For this review, take the finished solid that the model builds, in its own axes (mm). A direction names the side the tool comes from. Coordinates: 2 decimals unless noted, no trailing zeros. Loops run counter-clockwise (first coordinate to the right, second up) from the corner with the lowest first, then second, coordinate; pieces in that order, holes last. Notation, with made-up numbers: M 43.25,84.5 L 101.25,84.5 A22 cw 101.25,107.5 Z; hole C -26,-15 d7. An arc over 180 degrees is marked long. Answer as a JSON object with one key per item and string values. Group by question number.
Item 1: Add section D-D (x = 3.5). State the section outline as (y, z) points, then the cut area to 3 significant figures.
Item 2: Insertion check: pin 1 (10 mm diameter, centred on y = -0.5, z = 0, fed in from +X); pin 2 (1 mm diameter, centred on x = 3, z = -6, fed in from -Y); pin 3 (3 mm diameter, centred on x = 6, y = 1, fed in from -Z); pin 4 (1.9 mm diameter, centred on x = 5.5, y = 0, fed in from -Z). Each pin has a flat end and moves straight along its axis. Give the tip position at first contact, or say it passes through.
Item 3: Add section C-C (z = 5.5). State the section outline as (x, y) points.
Item 4: Add section A-A (x = 5.5). State the section outline as (y, z) points, then the cut area to 3 significant figures.
Item 5: Add section B-B (y = 0). State the section outline as (x, z) points.
Item 6: Mouldability with a two-part tool opening along Y and no side actions: class faces 1 (the face through (1.5, -16.5, 0.1)), 2 (the face through (1, -17.5, 0)), 3 (the face through (7.4, 5.93, -5.49)), 4 (the face through (3.6, -0.1, 4.5)) as +Y half, -Y half, draft (parallel to the pull), parting line (faces both ways), or undercut.
Item 7: Wall thickness on L1, parallel to Z at x = 5, y = 2.5; L2, parallel to Y at x = 5.5, z = 6; L3, parallel to X at y = 13, z = 7: over which ranges is each line inside the solid? List them lowest first. Write a range as from..to.
Item 8: Tool access review of faces 5 (the face through (3.6, -0.1, -6.5)), 6 (the face through (5, 6.5, -6)), 7 (the face through (1.5, -15.5, 7.5)), 8 (the face through (3.6, -0.1, -4.5)), 9 (the face through (5, -6.5, 5)): name each direction out of +Z, -Z, +X, -X, +Y, -Y from which nothing blocks a thin tool from reaching the whole face with its end or side.
from build123d import *

# Parameters (mm, degrees)
F0_W     = 35
F0_H     = 17
F1_DEPTH = 2
F2_W     = 2
F2_H     = 13
F2_H_2   = 1
F3_DEPTH = 1
F4_W     = 13
F4_H     = 2
F5_DEPTH = 6
F7_D     = 3.2
F8_R     = 2


with BuildPart() as f1:
    # F0 (on Right) → F1 (new body)
    with BuildSketch(Plane.YZ):
        Rectangle(F0_W, F0_H)
    extrude(amount=F1_DEPTH)

    # F2 (on face) → F3 (cut)
    with BuildSketch(Plane.YZ.offset(2)):
        with Locations((-15.5, 0)):
            Rectangle(F2_W, F2_H)
        with Locations((-15.5, 7)):
            Rectangle(F2_W, F2_H_2)
        with Locations((-15.5, -7)):
            Rectangle(F2_W, F2_H_2)
    extrude(amount=-F3_DEPTH, mode=Mode.SUBTRACT)

    # F4 (on face) → F5 (join)
    with BuildSketch(Plane.YZ.offset(2)):
        with Locations((0, 5.5)):
            Rectangle(F4_W, F4_H)
        with Locations((0, -5.5)):
            Rectangle(F4_W, F4_H)
    extrude(amount=F5_DEPTH)

    # F7 (through all)
    with Locations(Plane.XY.offset(6.5)):
        with Locations((5.5, 0)):
            Hole(F7_D / 2)

    # F8
    f8_edges = [f1.edges().sort_by_distance(p)[0] for p in [
        (2, 6.5, 5.5),
        (8, 6.5, 5.5),
        (8, 6.5, -5.5),
        (2, 6.5, -5.5),
        (2, -6.5, -5.5),
        (8, -6.5, -5.5),
        (2, -6.5, 5.5),
        (8, -6.5, 5.5),
    ]]
    fillet(f8_edges, radius=F8_R)


solid = f1.part
From the geometry:
{
 "1": {"outline": "M -6.56,-6.5 L 6.56,-6.5 L 6.56,-4.5 L -6.56,-4.5 Z; M -6.56,4.5 L 6.56,4.5 L 6.56,6.5 L -6.56,6.5 Z", "area": "52.5 mm²"},
 "2": {"pin 1": "stops at x = 8", "pin 2": "stops at y = -7.18", "pin 3": "stops at z = -6.5", "pin 4": "passes through"},
 "3": {"outline": "M 0,-17.5 L 2,-17.5 L 2,-16.5 L 1,-16.5 L 1,-14.5 L 2,-14.5 L 2,-8.5 A2 cw 4,-6.5 L 6,-6.5 A2 ccw 8,-4.5 L 8,4.5 A2 ccw 6,6.5 L 4,6.5 A2 cw 2,8.5 L 2,17.5 L 0,17.5 Z; hole C 5.5,0 d3.2"},
 "4": {"outline": "M -6.5,-6.5 L -1.6,-6.5 L -1.6,-4.5 L -6.5,-4.5 Z; M -6.5,4.5 L -1.6,4.5 L -1.6,6.5 L -6.5,6.5 Z; M 1.6,-6.5 L 6.5,-6.5 L 6.5,-4.5 L 1.6,-4.5 Z; M 1.6,4.5 L 6.5,4.5 L 6.5,6.5 L 1.6,6.5 Z", "area": "39.2 mm²"},
 "5": {"outline": "M 0,-8.5 L 2,-8.5 L 2,-6.5 L 3.9,-6.5 L 3.9,-4.5 L 2,-4.5 L 2,4.5 L 3.9,4.5 L 3.9,6.5 L 2,6.5 L 2,8.5 L 0,8.5 Z; M 7.1,-6.5 L 8,-6.5 L 8,-4.5 L 7.1,-4.5 Z; M 7.1,4.5 L 8,4.5 L 8,6.5 L 7.1,6.5 Z"},
 "6": {"face 1": "undercut", "face 2": "-Y half", "face 3": "+Y half", "face 4": "draft"},
 "7": {"L1": "z = -6.5..-4.5, 4.5..6.5", "L2": "y = -6.5..-1.6, 1.6..6.5", "L3": "x = 0..2"},
 "8": {"face 5": "-Z, +X, +Y, -Y", "face 6": "+Z, -Z, +X, +Y", "face 7": "+X", "face 8": "+X, +Y, -Y", "face 9": "+Z, -Z, +X, -Y"}
}
